Autodesk Inventor part; units mm, degrees
ref_plane "Work Plane1" through (12.5, 0, 0) normal (1, 0, 0) x (0, 1, 0)
ref_plane "XZ Plane" through (0, 0, 0) normal (0, 1, 0) x (-1, 0, 0)
ref_plane "XY Plane" through (0, 0, 0) normal (0, 0, 1) x (1, 0, 0)
sketch "Sketch1" plane through (0, 0, 0) normal (0, 1, 0) x (-1, 0, 0)
  circle A0 centre (0, 0) radius 7.5
  circle A1 centre (0, 0) radius 3
  dimension "d0" = 15
  dimension "d1" = 6
extrude "Extrusion1" add sketch "Sketch1" along normal blind 14
sketch "Sketch2" plane through (0, 14, 0) normal (0, 1, 0) x (1, 0, 0)
  circle A0 centre (0, 0) radius 3
  circle A1 centre (0, 0) radius 2.75
  circle A2 centre (0, 0) radius 4
  dimension "d4" = 5.5
  dimension "d5" = 8
extrude "Extrusion2" add sketch "Sketch2" along normal blind 7 contours A2
fillet "Fillet1" radius 6 1 edges at (-4, 14, 0)
fillet "Fillet2" radius 6 2 edges at (0, 14, -7.5) (0, 14, 7.5)
ref_plane "Work Plane1" through (12.5, 0, 0) normal (1, 0, 0) x (0, 1, 0)
mirror "Mirror1" about plane through (12.5, 0, 0) normal (1, 0, 0) of "Extrusion1", "Extrusion2", "Fillet1", "Fillet2"
sketch "Sketch3" plane through (0, 0, 0) normal (0, 1, 0) x (-1, 0, 0)
  circle A0 centre (-25, 0) radius 3
  line L0 (-25, 0) -> (-25, 3)
  line L1 (-25, 0) -> (-25, -3)
  line L2 (0, 0) -> (0, -3)
  circle A1 centre (0, 0) radius 3
  line L3 (0, 0) -> (0, 3)
  line L4 (-25, 3) -> (0, 3)
  line L5 (0, 3) -> (0, 7.5)
  line L6 (0, 7.5) -> (-25, 7.5)
  line L7 (-25, 7.5) -> (-25, 3)
  line L8 (-25, -3) -> (0, -3)
  line L9 (0, -3) -> (0, -7.5)
  line L10 (0, -7.5) -> (-25, -7.5)
  line L11 (-25, -7.5) -> (-25, -3)
  point P0 (0, -3)
  point P1 (0, 3)
  dimension "d11" = 25
  dimension "d12" = 4.5
  dimension "d13" = 25
  dimension "d14" = 4.5
extrude "Extrusion3" add sketch "Sketch3" along normal blind 11 contours A0 L4 A1 L8 | L7 L6 L5 L4 | L8 L9 L10 L11
sketch "Sketch4" plane through (0, 0, 7.5) normal (0, 0, 1) x (1, 0, 0)
  line L0 (25, 11) -> (0, 11)
  circle A0 centre (12.5, 5) radius 3
  line L1 (0, 0) -> (25, 0)
  line L2 (0, 0) -> (0, 10.9838)
  dimension "d18" = 6
  dimension "d21" = 5
  dimension "d22" = 12.5
extrude "Extrusion4" cut sketch "Sketch4" against normal through all
properties part number "4mm_Roller_Spacer_simple"
Source: CAD feature listing. Evaluate the final solid. Frame: model axes, mm. A direction names the side the tool comes from. Round coordinates to 2 decimals unless told otherwise and drop trailing zeros. Order: outer loops, then holes, each group sorted by start corner. A loop starts at its lowest first (then second) coordinate and runs counter-clockwise, first axis right, second up. Notation, with made-up numbers: (39.25, 7.5) - (74.25, 7.5) arc R22 cw to (74.25, 30.5) - close; hole circle Ø6 at (-15, 8.5). An arc over 180 degrees is marked (long way). Use a Markdown table: item, result. Add a question column.
1. Section query B-B (y = 7.5). Return the cut outline in (x, z).
2. Set-up query: faces 4 (the flat face through (10, 7, 7.5)), 5 (the cylindrical face through (-0.867, 20.216, -3.905)). Return all of +Z, -Z, +X, -X, +Y, -Y with unobstructed straight access to the full face (end or side cutting, diameter ignored); none if empty.
3. Section query C-C (z = -0.5). Give the number of separate pieces and of enclosed holes in the cut face, then the cut area to 3 significant figures.
4. Line query: probe 1 along Z at (x, y) = (0, 9.5); probe 2 along X at (y, z) = (2.75, 1); probe 3 along Y at (x, z) = (12.5, -2.5). Output: solid intervals per line, ascending.
5. Section query A-A (x = 12.5). Return the cut outline in (y, z), then the cut area to 3 significant figures.
6. Section query D-D (x = 17). Return the cut outline in (y, z), then the cut area to 3 significant figures.
7. First-contact query: pin 1 (1.5 mm diameter, centred on y = 4.5, z = -1, fed in from -X); pin 2 (1 mm diameter, centred on x = -3.5, y = 3.5, fed in from -Z). Flat tips, straight axial feed; report the tip coordinate or a pass-through.
8. Mould query, pull axis Z, two halves, no side actions, for faces 1 (the flat face through (13, 11, 0)), 2 (the flat face through (10, 7, -7.5)), 3 (the cylindrical face through (25, 10, 3)). Classes: +Z half, -Z half, draft (parallel to the pull), parting line (faces both ways), or undercut.
Derived:
| question | item | result |
|---|---|---|
| 1 | outline | (0, -7.5) - (10.84, -7.5) - (10.84, 7.5) - (0, 7.5) arc R7.5 ccw to start; (14.16, -7.5) - (25, -7.5) arc R7.5 ccw to (25, 7.5) - (14.16, 7.5) - close; hole circle Ø6 at (0, 0); hole circle Ø6 at (25, 0) |
| 2 | face 4 | +Z, +X, -X, +Y, -Y |
| 2 | face 5 | +Y |
| 3 | separate pieces | 3 |
| 3 | enclosed holes | 1 |
| 3 | area | 381 mm2 |
| 4 | probe 1 | -7.5 to -3, 3 to 7.5 |
| 4 | probe 2 | -7.43 to -2.83, 2.83 to 10.52, 14.48 to 22.17, 27.83 to 32.43 |
| 4 | probe 3 | 0 to 2, 8 to 11 |
| 5 | outline | (0, -7.5) - (2, -7.5) - (2, 7.5) - (0, 7.5) - close; (8, -7.5) - (11, -7.5) - (11, 7.5) - (8, 7.5) - close |
| 5 | area | 75.0 mm2 |
| 6 | outline | (0, -7.5) - (11, -7.5) - (11, 7.5) - (0, 7.5) - close |
| 6 | area | 165 mm2 |
| 7 | pin 1 | x = -7.5 |
| 7 | pin 2 | z = -6.87 |
| 8 | face 1 | draft |
| 8 | face 2 | -Z half |
| 8 | face 3 | undercut |
